Source: CAD feature listing. Evaluate the final solid. Frame: model axes, mm. A direction names the side the tool comes from. Round coordinates to 2 decimals unless told otherwise and drop trailing zeros. Write each loop counter-clockwise with the first axis right and the second up, starting at its lowest first coordinate (ties: lowest second). Pieces come first, ordered by that corner, then holes.
from build123d import *

# Parameters (mm, degrees)
SKETCH1_R           = 2.65
BOSS_EXTRUDE1_DEPTH = 16
SKETCH3_W           = 12.283798513
SKETCH3_H           = 21.086734885
CUT_EXTRUDE2_DEPTH  = 10
BOSS_EXTRUDE2_REACH = 32.583
SKETCH4_R           = 2


with BuildPart() as part:
    # Sketch1 → Boss-Extrude1 (new body)
    with BuildSketch(Plane.XY):
        with BuildLine():
            Line((0, 8), (-22, 2.922544759))
            ThreePointArc((-22, 2.922544759), (-24.325354345, -0.000692743), (-21.999845251, -2.923807139))
            Line((-21.999845251, -2.923807139), (0, -8))
            Line((0, -8), (21.999845251, -2.923807139))
            ThreePointArc((21.999845251, -2.923807139), (24.325354345, -0.000692743), (22, 2.922544759))
            Line((22, 2.922544759), (0, 8))
        make_face()
        with Locations((10, 0)):
            Circle(SKETCH1_R, mode=Mode.SUBTRACT)
        with Locations((-10, 0)):
            Circle(SKETCH1_R, mode=Mode.SUBTRACT)
    extrude(amount=BOSS_EXTRUDE1_DEPTH)

    # Sketch3 → Cut-Extrude2 (cut)
    with BuildSketch(Plane.XY.offset(16)):
        with Locations((0.115880044, 2.543367443)):
            Rectangle(SKETCH3_W, SKETCH3_H)
    extrude(amount=-CUT_EXTRUDE2_DEPTH, mode=Mode.SUBTRACT)

    # Sketch4 → Boss-Extrude2 (add, up to next)
    with BuildSketch(Plane.ZY.offset(-6.257779301), mode=Mode.PRIVATE) as boss_extrude2_sk1:
        with Locations((12, 0.000745713)):
            Circle(SKETCH4_R)
    boss_extrude2_tool1 = extrude(boss_extrude2_sk1.sketch, amount=BOSS_EXTRUDE2_REACH, mode=Mode.PRIVATE) - part.part
    add(boss_extrude2_tool1.solids().sort_by_distance((6.257779, 0.000746, 12))[0])


solid = part.part
1) Section query A-A on z = 9.5. Return the cut outline in (x, y).
Taken from the geometry:
outline: (-22, -2.92) - (-6.03, -6.61) - (-6.03, 6.61) - (-22, 2.92) arc R3 ccw to start; (6.26, -6.56) - (22, -2.92) arc R3 ccw to (22, 2.92) - (6.26, 6.56) - close; hole circle Ø5.3 at (-10, 0); hole circle Ø5.3 at (10, 0)
2) Section query C-C on x = 8. Return the cut outline in (y, z).
Taken from the geometry:
outline: (-6.15, 0) - (-1.74, 0) - (-1.74, 16) - (-6.15, 16) - close; (1.74, 0) - (6.15, 0) - (6.15, 16) - (1.74, 16) - close
3) Material intervals for line 1 (X direction, y = 1.75, z = 4.25); line 2 (X direction, y = 1.75, z = 14.75); line 3 (X direction, y = 0.25, z = 11.75), sorted ascending.
Taken from the geometry:
line 1: x = -23.76 to -11.99, -8.01 to 8.01, 11.99 to 23.76
line 2: x = -23.76 to -11.99, -8.01 to -6.03, 6.26 to 8.01, 11.99 to 23.76
line 3: x = -24.31 to -12.64, -7.36 to 7.36, 12.64 to 24.31
4) Reachability of faces 1 (the face through (0, 0, 0)), 2 (the face through (0, 0, 10)), 3 (the face through (0, 0, 6)) from +Z, -Z, +X, -X, +Y, -Y: full face, straight path, thin tool, end or side. Return the list, or none.
Taken from the geometry:
face 1: -Z, +X, -X, +Y, -Y
face 2: none
face 3: +Y, -Y
5) Pull-direction query (Y, two-part tool) for faces 4 (the face through (-13, 5, 8)), 5 (the face through (7.353, 0.117, 7.888)), 6 (the face through (6.258, -2, 10)); classes: released by +Y, released by -Y, zero draft, split by the parting line, or undercut.
Taken from the geometry:
face 4: released by +Y
face 5: undercut
face 6: zero draft
6) Section query D-D on y = -6. Return the cut outline in (x, z).
Taken from the geometry:
outline: (-8.67, 0) - (8.67, 0) - (8.67, 16) - (6.26, 16) - (6.26, 6) - (-6.03, 6) - (-6.03, 16) - (-8.67, 16) - close
7) Section query B-B on z = 2. Return the cut outline in (x, y), then the cut area to 3 significant figures.
Taken from the geometry:
outline: (-22, -2.92) - (0, -8) - (22, -2.92) arc R3 ccw to (22, 2.92) - (0, 8) - (-22, 2.92) arc R3 ccw to start; hole circle Ø5.3 at (-10, 0); hole circle Ø5.3 at (10, 0)
area: 457 mm2
8) Contact query for flat-ended pins moving along their axis: P1, Ø6, axis at y = 0.5, z = 3.5, coming from the +X side; P2, Ø1.5, axis at y = -3.5, z = 7.5, coming from the +X side; P3, Ø8, axis at x = 12, z = 3.5, coming from the -Y side; P4, Ø1, axis at x = -4.5, y = 3, coming from the +Z side. Output: stop coordinate, or through.
Taken from the geometry:
P1: stops at x = 24.33
P2: stops at x = 22.53
P3: stops at y = -6.15
P4: stops at z = 6
